Model file for the job. Use its own axes, mm. A direction names the side the tool comes from. Coordinates: 2 decimals unless noted, no trailing zeros. Loops run counter-clockwise (first coordinate to the right, second up) from the corner with the lowest first, then second, coordinate; pieces in that order, holes last. Notation, with made-up numbers: (-7.5, 47) -> (14.5, 47) arc R21 ccw to (14.5, 63) -> close; hole circle Ø7 at (-16.75, -38). An arc over 180 degrees is marked (long way). Use one line per item in the form item = value.
Autodesk Inventor part; units mm, degrees
ref_plane "YZ Plane" through (0, 0, 0) normal (1, 0, 0) x (0, 1, 0)
ref_plane "XZ Plane" through (0, 0, 0) normal (0, 1, 0) x (-1, 0, 0)
ref_plane "XY Plane" through (0, 0, 0) normal (0, 0, 1) x (1, 0, 0)
sketch "Sketch1" plane through (0, 0, 0) normal (0, 1, 0) x (-1, 0, 0)
  line L0 (0, 80) -> (0, 62.5) construction
  circle A0 centre (0, 62.5) radius 4
  line L1 (0, 62.5) -> (0, 0) construction
  circle A1 centre (-31.25, 54.1266) radius 4
  circle A2 centre (-54.1266, 31.25) radius 4
  circle A3 centre (-62.5, 0) radius 4
  circle A4 centre (-54.1266, -31.25) radius 4
  circle A5 centre (-31.25, -54.1266) radius 4
  circle A6 centre (0, -62.5) radius 4
  circle A7 centre (0, 0) radius 3.175
  line L2 (-78.5812, -15) -> (-95, -15)
  line L3 (-95, -15) -> (-95, 15)
  line L4 (-95, 15) -> (-78.5812, 15)
  line L5 (52.281, -60.5533) -> (60.4904, -74.7724)
  line L6 (60.4904, -74.7724) -> (34.5096, -89.7724)
  line L7 (34.5096, -89.7724) -> (26.3002, -75.5533)
  line L8 (26.3002, 75.5533) -> (34.5096, 89.7724)
  line L9 (34.5096, 89.7724) -> (60.4904, 74.7724)
  line L10 (60.4904, 74.7724) -> (52.281, 60.5533)
  arc A8 (52.281, -60.5533) -> (52.281, 60.5533) centre (0, 0) ccw
  arc A9 (26.3002, 75.5533) -> (-78.5812, 15) centre (0, 0) ccw
  arc A10 (-78.5812, -15) -> (26.3002, -75.5533) centre (0, 0) ccw
  point P0 (80, 0)
  dimension "d2" = 8
  dimension "d5" = 180
  dimension "d7" = 6.35
  dimension "d10" = 62.5
  dimension "d12" = 95
  dimension "d13" = 30
  dimension "d16" = 360
  dimension "d18" = 80
extrude "Extrusion1" add sketch "Sketch1" along normal blind 6
sketch "Sketch3" plane through (0, 6, 0) normal (0, 1, 0) x (1, 0, 0)
  line L0 (95, 15) -> (78.5812, 15)
  line L1 (78.5812, -15) -> (95, -15)
  line L2 (95, -15) -> (95, 15)
  point P0 (0, 0)
  point P1 (88, 8)
  point P2 (88, -8)
  point P3 (86.7906, -15)
  point P4 (-50.9282, 72.2102)
  point P5 (-37.0718, 80.2102)
  point P6 (-37.0718, -80.2102)
  point P7 (-50.9282, -72.2102)
  dimension "d19" = 7
  dimension "d20" = 7
  dimension "d21" = 7
  dimension "d24" = 360
hole "Hole1" at (88, 6, -8) at (88, 6, 8) at (-50.9282, 6, -72.2102) at (-37.0718, 6, -80.2102) at (-37.0718, 6, 80.2102) at (-50.9282, 6, 72.2102) direction (0, -1, 0) diameter 4.5 end through all
sketch "Sketch4" plane through (0, 6, 0) normal (0, 1, 0) x (1, 0, 0)
  circle A0 centre (0, 15) radius 2.5
  circle A1 centre (0, -15) radius 2.5
  circle A2 centre (0, 0) radius 3.175 construction
  line L0 (0, 0) -> (8.7984, 0) construction
  dimension "d33" = 5
  dimension "d34" = 15
extrude "Extrusion2" cut sketch "Sketch4" against normal blind 6
fillet "Fillet1" radius 2 12 edges at (-52.281, 3, 60.5533) (-60.4904, 3, 74.7724) (-34.5096, 3, 89.7724) (-26.3002, 3, 75.5533) (78.5812, 3, 15) (95, 3, 15) (95, 3, -15) (78.5812, 3, -15) (-26.3002, 3, -75.5533) (-34.5096, 3, -89.7724) (-52.281, 3, -60.5533) (-60.4904, 3, -74.7724)
properties part number "SkimmerLid"
Q1. Band-saw the part on A-A, the plane x = 0. Write the cut outline in (y, z) (3 decimals).
Result:
outline = (0, -80) -> (6, -80) -> (6, -66.5) -> (0, -66.5) -> close; (0, -58.5) -> (6, -58.5) -> (6, -17.5) -> (0, -17.5) -> close; (0, -12.5) -> (6, -12.5) -> (6, -3.175) -> (0, -3.175) -> close; (0, 3.175) -> (6, 3.175) -> (6, 12.5) -> (0, 12.5) -> close; (0, 17.5) -> (6, 17.5) -> (6, 58.5) -> (0, 58.5) -> close; (0, 66.5) -> (6, 66.5) -> (6, 80) -> (0, 80) -> close
Q2. Wall check: line 1 along Z through (x, y) = (0, 2.7) (3 decimals); line 2 along Z through (x, y) = (57, 3); line 3 along X through (y, z) = (5.2, -2). Give the ranges that are in metal, low to high.
Result:
line_1 = -80 to -66.5, -58.5 to -17.5, -12.5 to -3.175, 3.175 to 12.5, 17.5 to 58.5, 66.5 to 80
line_2 = -56.13 to -34.03, -28.47 to 28.47, 34.03 to 56.13
line_3 = -79.98 to -2.47, 2.47 to 59.04, 65.96 to 95
Q3. Which spindle directions (+Z, -Z, +X, -X, +Y, -Y) get a long thin tool onto all of the face, cutting with end or side? Do faces 1 (the face through (-30.359, 2.958, -82.583)), 2 (the face through (-30.27, 2.96, 82.43)), 3 (the face through (-35.076, 2.958, 81.248)), 4 (the face through (-56.34, 2.96, 67.58)). Say none if no direction does.
Result:
face_1 = -Z, +Y, -Y
face_2 = +Z, +Y, -Y
face_3 = +Y, -Y
face_4 = -X, +Y, -Y
Q4. Mould opens along Z. For faces 5 (the face through (9, 0, 1)), 6 (the face through (57.075, 2.958, -33.953)), 7 (the face through (-47.66, 2.96, -82.18)) say: released by +Z, released by -Z, zero draft, split by the parting line, or undercut.
Result:
face_5 = zero draft
face_6 = undercut
face_7 = released by -Z
Q5. Band-saw the part on D-D, the plane z = 31.25. Write the cut outline in (x, y), and give its area (3 significant figures).
Result:
outline = (-73.64, 0) -> (50.13, 0) -> (50.13, 6) -> (-73.64, 6) -> close; (58.13, 0) -> (73.64, 0) -> (73.64, 6) -> (58.13, 6) -> close
area = 836 mm2
Q6. Pin check, flat tips, straight feed: pin 1 Ø2.5 at (x, z) = (-50.93, 72.21) entering from +Y; pin 2 Ø1.5 at (y, z) = (4, 27) entering from -X; pin 3 Ø2 at (x, y) = (-10.5, 5) entering from -Z. Stop position of each tip, or through.
Result:
pin_1 = through
pin_2 = -75.57
pin_3 = -79.43
Q7. Band-saw the part on C-C, the plane x = -56.5. Write the cut outline in (y, z).
Result:
outline = (0, -77.08) -> (6, -77.08) -> (6, -67.86) -> (0, -67.86) -> close; (0, -56.64) -> (6, -56.64) -> (6, 56.64) -> (0, 56.64) -> close; (0, 67.86) -> (6, 67.86) -> (6, 77.08) -> (0, 77.08) -> close
Q8. Band-saw the part on B-B, the plane z = -8. Write the cut outline in (x, y).
Result:
outline = (-79.6, 0) -> (85.75, 0) -> (85.75, 6) -> (-79.6, 6) -> close; (90.25, 0) -> (95, 0) -> (95, 6) -> (90.25, 6) -> close
